Part model, mm, in its own coordinate system. A direction names the side the tool comes from. Give positions to 0.01 mm unless a question says otherwise; leave off trailing zeros. Order: outer loops, then holes, each group sorted by start corner. A loop starts at its lowest first (then second) coordinate and runs counter-clockwise, first axis right, second up. Notation, with made-up numbers: M -9.5,73 L 26.5,73 A13 ccw 26.5,93 Z; hole C -34,-24 d3. An arc over 180 degrees is marked long. Return JSON: item names as keys, results as strings.
from build123d import *

# Parameters (mm, degrees)
F2_R    = 5.08
F3_SIZE = 5.08


with BuildPart() as f1:
    # F0 (on Front) → F1 (revolve)
    with BuildSketch(Plane.XZ):
        Polygon((0, 55.314001), (0, 13.251298), (11.915691, 13.251298), (11.915691, 20.03995), (15.310015, 20.03995), (38.080281, 46.34597), (38.080281, 55.314001), align=None)
    revolve(axis=Axis((25.323285, 0, 0), (1, 0, 0)))

    # F2
    f2_edges = [f1.edges().sort_by_distance(p)[0] for p in [
        (38.080281, 0, -46.34597),
        (38.080281, 0, -55.314001),
    ]]
    fillet(f2_edges, radius=F2_R)

    # F3
    f3_edges = [f1.edges().sort_by_distance(p)[0] for p in [
        (0, 0, -55.314001),
    ]]
    chamfer(f3_edges, length=F3_SIZE)


solid = f1.part
Q1. 3-axis set-ups, long thin cutter, end or side, ignore diameter. For faces 4 (the flat face through (0, 10, 10)), 5 (the cylindrical face through (13.6, 12.2, -15.9)): which of +Z, -Z, +X, -X, +Y, -Y reach the whole face in a straight line?
Established:
{"face 4": "+Z, -Z, -X, +Y, -Y", "face 5": "+X"}
Q2. Two-plate mould, pull along Y, no slides. Class faces 1 (the conical face through (0.247, 49.28, -10.943)), 2 (the cylindrical face through (6.04, -3.98, 12.64)), 3 (the flat face through (38.08, -45, 19)): +Y half, -Y half, draft (parallel to the pull), parting line (faces both ways), or undercut.
Established:
{"face 1": "parting line", "face 2": "undercut", "face 3": "draft"}
Q3. Pin check, flat tips, straight feed: pin 1 (3 mm diameter, centred on x = 22, z = 43.5, fed in from +Y) (3 decimals); pin 2 (1.5 mm diameter, centred on x = 28, z = 3.5, fed in from +Y); pin 3 (1.5 mm diameter, centred on y = -40, z = -20, fed in from +X); pin 4 (24 mm diameter, centred on y = 0, z = 0, fed in from +X). Stop position of each tip, or through.
Established:
{"pin 1": "stops at y = 35.995", "pin 2": "stops at y = 55.25", "pin 3": "stops at x = 37.26", "pin 4": "passes through"}
Q4. Band-saw the part on A-A (z = 0). Give the cut face in (x, y).
Established:
{"outline": "M 0,-50.23 L 5.08,-55.31 L 33,-55.31 A5.08 ccw 38.08,-50.23 L 38.08,-48.24 A5.08 ccw 36.84,-44.91 L 15.31,-20.04 L 11.92,-20.04 L 11.92,-13.25 L 0,-13.25 Z; M 0,13.25 L 11.92,13.25 L 11.92,20.04 L 15.31,20.04 L 36.84,44.91 A5.08 ccw 38.08,48.24 L 38.08,50.23 A5.08 ccw 33,55.31 L 5.08,55.31 L 0,50.23 Z"}
Q5. Band-saw the part on D-D (x = 28). Give the cut face in (y, z), then the cut area to 3 significant figures.
Established:
{"outline": "C 0,0 d110.63; hole C 0,0 d69.4", "area": "5,830 mm²"}
Q6. Band-saw the part on C-C (x = 19). Give the cut face in (y, z), then the cut area to 3 significant figures.
Established:
{"outline": "C 0,0 d110.63; hole C 0,0 d48.61", "area": "7,760 mm²"}
Q7. Probe line 1 along Y through (x, z) = (14, 0); line 2 along Y through (x, z) = (6.5, 0). List the from-to ranges inside material, lowest first.
Established:
{"line 1": "y = -55.31 to -20.04, 20.04 to 55.31", "line 2": "y = -55.31 to -13.25, 13.25 to 55.31"}
